from build123d import *

# Parameters (mm, degrees)
SKETCH1_W           = 62.46
SKETCH1_H           = 18
BOSS_EXTRUDE1_DEPTH = 3
SKETCH2_W           = 22.3
SKETCH2_H           = 3
SKETCH2_W_2         = 22.29
SKETCH2_W_3         = 26.23
CUT_EXTRUDE1_DEPTH  = 3
FILLET1_R           = 2
FILLET2_R           = 2


with BuildPart() as part:
    # Sketch1 → Boss-Extrude1 (new body)
    with BuildSketch(Plane.XY):
        Rectangle(SKETCH1_W, SKETCH1_H)
    extrude(amount=BOSS_EXTRUDE1_DEPTH)

    # Sketch2 → Cut-Extrude1 (cut)
    with BuildSketch(Plane.XY.offset(3)):
        with Locations((20.08, -7.5)):
            Rectangle(SKETCH2_W, SKETCH2_H)
        with Locations((-20.085, -7.5)):
            Rectangle(SKETCH2_W_2, SKETCH2_H)
        with Locations((18.115, 7.5)):
            Rectangle(SKETCH2_W_3, SKETCH2_H)
        with Locations((-18.115, 7.5)):
            Rectangle(SKETCH2_W_3, SKETCH2_H)
    extrude(amount=-CUT_EXTRUDE1_DEPTH, mode=Mode.SUBTRACT)

    # Fillet1
    fillet1_edges = [part.edges().sort_by_distance(p)[0] for p in [
        (31.23, 0, 3),
    ]]
    fillet(fillet1_edges, radius=FILLET1_R)

    # Fillet2
    fillet2_edges = [part.edges().sort_by_distance(p)[0] for p in [
        (-31.23, 0, 3),
    ]]
    fillet(fillet2_edges, radius=FILLET2_R)


solid = part.part
The model under review builds one solid part; all positions refer to its coordinate system, in mm. A direction names the side the tool comes from. Round coordinates to 2 decimals unless told otherwise and drop trailing zeros. Write each loop counter-clockwise with the first axis right and the second up, starting at its lowest first coordinate (ties: lowest second). Pieces come first, ordered by that corner, then holes. Notation, with made-up numbers: (56.5, 35.25) -> (65.5, 35.25) arc R30 cw to (65.5, 64.25) -> close; hole circle Ø3 at (22.5, 39). An arc over 180 degrees is marked (long way). Answer as a JSON object with one key per item and string values.
1. Clearance check with flat-ended pins moving along their axes: pin 1 (1.5 mm diameter, centred on y = -7, z = 1.5, fed in from +X); pin 2 (0.9 mm diameter, centred on x = -22.5, z = 2, fed in from -Y). State where each tip first meets the part, or that it passes through.
Results found:
{"pin 1": "stops at x = 8.93", "pin 2": "stops at y = -6"}
2. Machinability: for faces 1 (the face through (30.63, 0.08, 2.43)), 2 (the face through (-20, -6, 2)), 3 (the face through (20, -6, 2)), 4 (the face through (-18, 6, 2)), 5 (the face through (18, 6, 2)), which of the approach directions +Z, -Z, +X, -X, +Y, -Y give a long, thin tool a straight path to every point of the face, cutting with its end or side? Answer none if there is none.
Results found:
{"face 1": "+Z, +X, +Y, -Y", "face 2": "+Z, -Z, -X, -Y", "face 3": "+Z, -Z, +X, -Y", "face 4": "+Z, -Z, -X, +Y", "face 5": "+Z, -Z, +X, +Y"}
3. We need section B-B on x = -18.5. State the section outline as (y, z) points, and give its area (3 significant figures).
Results found:
{"outline": "(-6, 0) -> (6, 0) -> (6, 3) -> (-6, 3) -> close", "area": "36.0 mm^2"}
4. To check wall thickness, follow line 1 along Y through (x, z) = (-22.5, 2.8); line 2 along X through (y, z) = (-6.5, 2.7); line 3 along Y through (x, z) = (8.5, 0.7). State the ranges of each line that lie inside material, in increasing order.
Results found:
{"line 1": "y = -6 to 6", "line 2": "x = -8.94 to 8.93", "line 3": "y = -9 to 6"}
5. We need section C-C on y = 7.5. State the section outline as (x, z) points.
Results found:
{"outline": "(-5, 0) -> (5, 0) -> (5, 3) -> (-5, 3) -> close"}
6. We need section A-A on z = 0.55. State the section outline as (x, y) points, and give its area (3 significant figures).
Results found:
{"outline": "(-31.23, -6) -> (-8.94, -6) -> (-8.94, -9) -> (8.93, -9) -> (8.93, -6) -> (31.23, -6) -> (31.23, 6) -> (5, 6) -> (5, 9) -> (-5, 9) -> (-5, 6) -> (-31.23, 6) -> close", "area": "833 mm^2"}
